from build123d import *

# Parameters (mm, degrees)
SKETCH1_R           = 1.1
BOSS_EXTRUDE1_DEPTH = 6.35
FILLET1_R           = 5


with BuildPart() as part:
    # Sketch1 → Boss-Extrude1 (new body)
    with BuildSketch(Plane.XY):
        with BuildLine():
            Line((-30.671332299, 7.5), (-26.768089678, 10))
            ThreePointArc((-26.768089678, 10), (0, 28.575), (26.768089678, 10))
            Line((26.768089678, 10), (30.671332299, 7.5))
            ThreePointArc((30.671332299, 7.5), (31.575, 0), (30.671332299, -7.5))
            Line((30.671332299, -7.5), (26.768089678, -10))
            ThreePointArc((26.768089678, -10), (0, -28.575), (-26.768089678, -10))
            Line((-26.768089678, -10), (-30.671332299, -7.5))
            ThreePointArc((-30.671332299, -7.5), (-31.575, 0), (-30.671332299, 7.5))
        make_face()
        with Locations((-25.4, 0)):
            Circle(SKETCH1_R, mode=Mode.SUBTRACT)
        with Locations((-12.7, 21.997045256)):
            Circle(SKETCH1_R, mode=Mode.SUBTRACT)
        with Locations((12.7, 21.997045256)):
            Circle(SKETCH1_R, mode=Mode.SUBTRACT)
        with Locations((25.4, 0)):
            Circle(SKETCH1_R, mode=Mode.SUBTRACT)
        with Locations((12.7, -21.997045256)):
            Circle(SKETCH1_R, mode=Mode.SUBTRACT)
        with Locations((-12.7, -21.997045256)):
            Circle(SKETCH1_R, mode=Mode.SUBTRACT)
    extrude(amount=BOSS_EXTRUDE1_DEPTH)

    # Fillet1
    fillet1_edges = [part.edges().sort_by_distance(p)[0] for p in [
        (30.671332299, -7.5, 3.175),
        (26.768089678, -10, 3.175),
        (-26.768089678, -10, 3.175),
        (-30.671332299, -7.5, 3.175),
        (-30.671332299, 7.5, 3.175),
        (-26.768089678, 10, 3.175),
        (26.768089678, 10, 3.175),
        (30.671332299, 7.5, 3.175),
    ]]
    fillet(fillet1_edges, radius=FILLET1_R)


solid = part.part
The listing builds one solid part. Answer for the finished solid, in the listing's coordinates (mm). Give positions to 0.01 mm unless a question says otherwise; leave off trailing zeros. Write each loop counter-clockwise with the first axis right and the second up, starting at its lowest first coordinate (ties: lowest second). Pieces come first, ordered by that corner, then holes. Notation, with made-up numbers: (73, 56.5) - (96, 56.5) arc R24 ccw to (96, 89.5) - close; hole circle Ø6 at (35, 16.25). An arc over 180 degrees is marked (long way). Use a Markdown table: item, result.
1. Section B-B on x = 25.4 is taken. Write down the section's boundary in (y, z), plus the area to 3 significant figures.
Values follow:
| item | result |
|---|---|
| outline | (-13.09, 0) - (-1.1, 0) - (-1.1, 6.35) - (-13.09, 6.35) - close; (1.1, 0) - (13.09, 0) - (13.09, 6.35) - (1.1, 6.35) - close |
| area | 152 mm² |
2. Find the intervals of material crossed by probe 1 along X at (y, z) = (-22.5, 3.5); probe 2 along Y at (x, z) = (-12.7, 2.5); probe 3 along X at (y, z) = (21.5, 0.5), in increasing order. Write a range as from..to.
Values follow:
| item | result |
|---|---|
| probe 1 | x = -17.61..-13.68, -11.72..11.72, 13.68..17.61 |
| probe 2 | y = -25.6..-23.1, -20.9..20.9, 23.1..25.6 |
| probe 3 | x = -18.82..-13.68, -11.72..11.72, 13.68..18.82 |
3. Section D-D on x = -12.7 is taken. Write down the section's boundary in (y, z), plus the area to 3 significant figures.
Values follow:
| item | result |
|---|---|
| outline | (-25.6, 0) - (-23.1, 0) - (-23.1, 6.35) - (-25.6, 6.35) - close; (-20.9, 0) - (20.9, 0) - (20.9, 6.35) - (-20.9, 6.35) - close; (23.1, 0) - (25.6, 0) - (25.6, 6.35) - (23.1, 6.35) - close |
| area | 297 mm² |
4. Each of these flat-tipped pins is pushed along its axis until it touches: P1, Ø4, axis at x = 5.5, y = 12.5, coming from the -Z side; P2, Ø1.3, axis at x = -25.4, y = 0, coming from the -Z side; P3, Ø1.5, axis at x = 24.5, z = 1, coming from the -Y side; P4, Ø1, axis at x = 17.5, z = 4.5, coming from the +Y side. Where does it stop, or does it pass through?
Values follow:
| item | result |
|---|---|
| P1 | stops at z = 0 |
| P2 | passes through |
| P3 | stops at y = -15.89 |
| P4 | stops at y = 22.97 |
5. Section A-A on y = 0 is taken. Write down the section's boundary in (x, z) (3 decimals).
Values follow:
| item | result |
|---|---|
| outline | (-31.575, 0) - (-26.5, 0) - (-26.5, 6.35) - (-31.575, 6.35) - close; (-24.3, 0) - (24.3, 0) - (24.3, 6.35) - (-24.3, 6.35) - close; (26.5, 0) - (31.575, 0) - (31.575, 6.35) - (26.5, 6.35) - close |
6. For a pull along Y with two mould halves and no side action, classify faces 1 (the flat face through (0, 0, 6.35)), 2 (the cylindrical face through (30.359, 7.205, 3.219)), 3 (the cylindrical face through (-12.84, 23.09, 3.13)) as released by +Y, released by -Y, zero draft, split by the parting line, or undercut.
Values follow:
| item | result |
|---|---|
| face 1 | zero draft |
| face 2 | released by +Y |
| face 3 | undercut |
7. Section C-C on z = 4.25 is taken. Count the separate pieces of the cut face and the enclosed holes in it, plus the area to 3 significant figures.
Values follow:
| item | result |
|---|---|
| separate pieces | 1 |
| enclosed holes | 6 |
| area | 2,650 mm² |
